The model under review builds one solid part; all positions refer to its coordinate system, in mm. Face numbers are marked on the shaded views. Round coordinates to 2 decimals unless told otherwise and drop trailing zeros. Order: outer loops, then holes, each group sorted by start corner. A loop starts at its lowest first (then second) coordinate and runs counter-clockwise, first axis right, second up. Notation, with made-up numbers: M 88.25,39 L 145.25,39 A7 ccw 145.25,52 Z; hole C 44,-40 d11. An arc over 180 degrees is marked long. Use a Markdown table: item, result. Add a question column.
1. Consider section B-B on z = 139. State the section outline as (x, y) points.
2. The part is to be moulded in two halves that separate along X. For the marked faces 1, 2, 3 and 4, say which applies: +X half, -X half, draft (parallel to the pull), parting line (faces both ways), or undercut.
3. Consider section A-A on z = 199. Count the separate pieces of the cut face and the enclosed holes in it, then the cut area to 3 significant figures.
4. Consider section D-D on y = 1.5. State the section outline as (x, z) points.
5. Consider section C-C on x = -63.5. State the section outline as (y, z) points (3 decimals).
6. To check wall thickness, follow probe 1 along Z at (x, y) = (88.9, -92.5); probe 2 along X at (y, z) = (-92, 209.55); probe 3 along X at (y, z) = (-84.5, 50.5). State the ranges of each line that lie inside material, in increasing order.
7. Insertion check: P1, Ø14, axis at x = -26.5, y = 83.5, coming from the +Z side; P2, Ø0.6, axis at x = -17.5, y = -88.5, coming from the +Z side; P3, Ø2.5, axis at x = 17, z = -1.5, coming from the -Y side; P4, Ø3, axis at x = -96.34, z = 209.55, coming from the +Y side. Each pin has a flat end and moves straight along its axis. Give the tip position at first contact, or say it passes through.
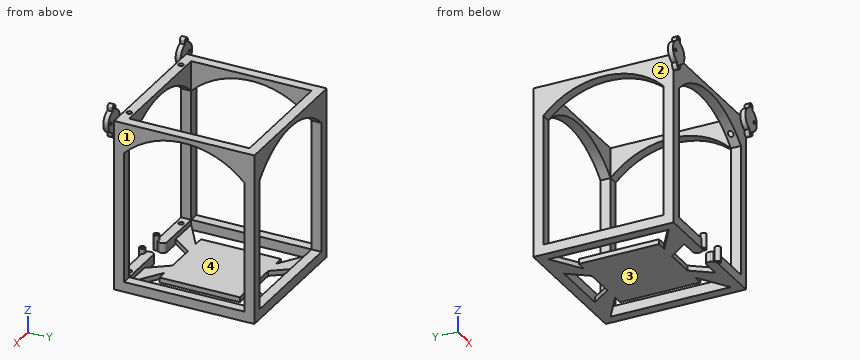
from build123d import *

# Parameters (mm, degrees)
F0_W      = 101.6
F0_H      = 101.6
F1_DEPTH  = 6.35
F2_W      = 12.7
F2_H      = 12.7
F3_DEPTH  = 88.9
F5_W      = 12.7
F5_H      = 12.7
F6_DEPTH  = 76.2
F9_W      = 38.1
F9_H      = 6.35
F8_W      = 19.05
F8_H      = 6.35
F14_W     = 12.7
F14_H     = 12.7
F15_DEPTH = 203.2
F17_DEPTH = 12.7
F20_DEPTH = 12.7
F22_R     = 3.175
F23_DEPTH = 209.55
F24_R     = 1.905
F24_R_2   = 1.778
F25_DEPTH = 19.05
F27_DEPTH = 25.4
F28_R     = 5.08
F29_R     = 1.778
F29_R_2   = 1.905
F30_DEPTH = 6.35


# Not quite as in the source:
# - a feature of the source that left no trace in its solid (it failed there, or was rolled back) is left out


with BuildPart() as f1:
    # F0 (on Top) → F1 (new body)
    with BuildSketch(Plane.XY):
        Rectangle(F0_W, F0_H)
    extrude(amount=-F1_DEPTH)



with BuildPart() as f3:
    # F2 (on Right) → F3 (new body, symmetric)
    with BuildSketch(Plane.YZ):
        with Locations((-82.55, 0)):
            Rectangle(F2_W, F2_H)
    extrude(amount=F3_DEPTH, both=True)


with BuildPart() as f4_1:
    # F4: instance of F3
    add(f3.part.mirror(Plane.XZ))


with BuildPart() as f3_1:
    add(f3.part)

    add(f4_1.part)  # F6 merges F4_1
    # F5 (on Front) → F6 (join, symmetric)
    with BuildSketch(Plane.XZ):
        with Locations((82.55, 0)):
            Rectangle(F5_W, F5_H)
    extrude(amount=F6_DEPTH, both=True)


with BuildPart() as f7_1:
    # F7: instance of F3
    add(f3_1.part.mirror(Plane.YZ))


with BuildPart() as f1_1:
    add(f1.part)

    add(f3_1.part)  # F10 merges F3

    add(f7_1.part)  # F10 merges F7_1
    # F9 (on face) → F10 section 0
    with BuildSketch(Plane(origin=(0, -76.2, 0), x_dir=(-1, 0, 0), z_dir=(0, 1, 0))):
        with Locations((57.15, -3.175)):
            Rectangle(F9_W, F9_H)
    # F8 (on face) → F10 section 1
    with BuildSketch(Plane.XZ.offset(50.8)):
        with Locations((-28.575, -3.175)):
            Rectangle(F8_W, F8_H)
    loft()


with BuildPart() as f11_1:
    # F11: instance of F1
    add(f1_1.part.mirror(Plane.YZ))


with BuildPart() as f12_1:
    # F12: instance of F11_1
    add(f11_1.part.mirror(Plane.XZ))


with BuildPart() as f12_2:
    # F12: instance of F1
    add(f1_1.part.mirror(Plane.XZ))


with BuildPart() as f1_2:
    add(f1_1.part)

    # F13: union F12_2, F11_1, F12_1
    add(f12_2.part)
    add(f11_1.part)
    add(f12_1.part)

    # F14 (on face) → F15 (join)
    with BuildSketch(Plane.XY.offset(6.35)):
        with Locations((-82.55, 82.55)):
            Rectangle(F14_W, F14_H)
        with Locations((82.55, 82.55)):
            Rectangle(F14_W, F14_H)
        with Locations((82.55, -82.55)):
            Rectangle(F14_W, F14_H)
        with Locations((-82.55, -82.55)):
            Rectangle(F14_W, F14_H)
    extrude(amount=F15_DEPTH)

    # F16 (on face) → F17 (join)
    with BuildSketch(Plane(origin=(-88.9, 0, 0), x_dir=(0, -1, 0), z_dir=(-1, 0, 0))):
        with BuildLine():
            ThreePointArc((-76.2, 171.45), (0, 203.2), (76.2, 171.45))
            Line((76.2, 171.45), (76.2, 209.55))
            Line((76.2, 209.55), (-76.2, 209.55))
            Line((-76.2, 209.55), (-76.2, 171.45))
        make_face()
    extrude(amount=-F17_DEPTH)

    # F18: F1 across plane


with BuildPart() as f1_3:
    add(f1_2.part)
    add(f1_2.part.mirror(Plane.YZ))

    # F19 (on face) → F20 (join)
    with BuildSketch(Plane(origin=(0, 88.9, 0), x_dir=(-1, 0, 0), z_dir=(0, 1, 0))):
        with BuildLine():
            ThreePointArc((-76.2, 171.45), (0, 203.2), (76.2, 171.45))
            Line((76.2, 171.45), (76.2, 209.55))
            Line((76.2, 209.55), (-76.2, 209.55))
            Line((-76.2, 209.55), (-76.2, 171.45))
        make_face()
    extrude(amount=-F20_DEPTH)

    # F21: F1 across plane


with BuildPart() as f1_4:
    add(f1_3.part)
    add(f1_3.part.mirror(Plane.XZ))

    # F22 (on face) → F23 (cut)
    with BuildSketch(Plane.XY.offset(209.55)):
        with Locations((-63.5, -82.55)):
            Circle(F22_R)
        with Locations((63.5, -82.55)):
            Circle(F22_R)
    extrude(amount=-F23_DEPTH, mode=Mode.SUBTRACT)

    # F24 (on face) → F25 (join)
    with BuildSketch(Plane(origin=(0, 0, -6.35), x_dir=(1, 0, 0), z_dir=(0, 0, -1))):
        with BuildLine():
            Line((17.45107, 93.48597), (13.5244245713, 93.48597))
            ThreePointArc((13.5244245713, 93.48597), (0, 103.95585), (-13.5244245713, 93.48597))
            Line((-13.5244245713, 93.48597), (-17.45107, 93.48597))
            ThreePointArc((-17.45107, 93.48597), (-20.95119, 89.98585), (-17.45107, 86.48573))
            Line((-17.45107, 86.48573), (-13.5244245713, 86.48573))
            ThreePointArc((-13.5244245713, 86.48573), (0, 76.01585), (13.5244245713, 86.48573))
            Line((13.5244245713, 86.48573), (17.45107, 86.48573))
            ThreePointArc((17.45107, 86.48573), (20.95119, 89.98585), (17.45107, 93.48597))
        make_face()
        with Locations((0, 82.55)):
            Circle(F24_R, mode=Mode.SUBTRACT)
        with Locations((-17.45107, 89.98585)):
            Circle(F24_R_2, mode=Mode.SUBTRACT)
        with Locations((17.45107, 89.98585)):
            Circle(F24_R_2, mode=Mode.SUBTRACT)
    extrude(amount=-F25_DEPTH)

    # F26 (on face) → F27 (cut)
    with BuildSketch(Plane.XY.offset(12.7)):
        with BuildLine():
            ThreePointArc((-17.45107, -86.48573), (-15.0942845585, -87.3981092098), (-13.9661895841, -89.6595855349))
            ThreePointArc((-13.9661895841, -89.6595855349), (-13.97, -89.98585), (-13.9661895841, -90.3121144651))
            ThreePointArc((-13.9661895841, -90.3121144651), (-15.0942845585, -92.5735907902), (-17.45107, -93.48597))
            Line((-17.45107, -93.48597), (-13.5244245713, -93.48597))
            ThreePointArc((-13.5244245713, -93.48597), (0, -103.95585), (13.5244245713, -93.48597))
            Line((13.5244245713, -93.48597), (17.45107, -93.48597))
            ThreePointArc((17.45107, -93.48597), (13.95095, -89.98585), (17.45107, -86.48573))
            Line((17.45107, -86.48573), (13.5244245713, -86.48573))
            ThreePointArc((13.5244245713, -86.48573), (0, -76.01585), (-13.5244245713, -86.48573))
            Line((-13.5244245713, -86.48573), (-17.45107, -86.48573))
        make_face()
    extrude(amount=-F27_DEPTH, mode=Mode.SUBTRACT)

    # F28
    f28_edges = [f1_4.edges().sort_by_distance(p)[0] for p in [
        (2.260805, -76.2, 0),
        (-2.260805, -76.2, 0),
    ]]
    fillet(f28_edges, radius=F28_R)

    # F29 (on face) → F30 (join)
    with BuildSketch(Plane.XZ.offset(88.9)):
        with BuildLine():
            Line((-85.39988, 192.09893), (-85.39988, 196.0255754287))
            ThreePointArc((-85.39988, 196.0255754287), (-74.93, 209.55), (-85.39988, 223.0744245713))
            Line((-85.39988, 223.0744245713), (-85.39988, 227.00107))
            ThreePointArc((-85.39988, 227.00107), (-88.9, 230.50119), (-92.40012, 227.00107))
            Line((-92.40012, 227.00107), (-92.40012, 223.0744245713))
            ThreePointArc((-92.40012, 223.0744245713), (-102.87, 209.55), (-92.40012, 196.0255754287))
            Line((-92.40012, 196.0255754287), (-92.40012, 192.09893))
            ThreePointArc((-92.40012, 192.09893), (-88.9, 188.59881), (-85.39988, 192.09893))
        make_face()
        with Locations((-88.9, 192.09893)):
            Circle(F29_R, mode=Mode.SUBTRACT)
        with Locations((-96.33585, 209.55)):
            Circle(F29_R_2, mode=Mode.SUBTRACT)
        with Locations((-88.9, 227.00107)):
            Circle(F29_R, mode=Mode.SUBTRACT)
        with BuildLine():
            Line((85.39988, 227.00107), (85.39988, 223.0744245713))
            ThreePointArc((85.39988, 223.0744245713), (74.93, 209.55), (85.39988, 196.0255754287))
            Line((85.39988, 196.0255754287), (85.39988, 192.09893))
            ThreePointArc((85.39988, 192.09893), (88.9, 188.59881), (92.40012, 192.09893))
            Line((92.40012, 192.09893), (92.40012, 196.0255754287))
            ThreePointArc((92.40012, 196.0255754287), (102.87, 209.55), (92.40012, 223.0744245713))
            Line((92.40012, 223.0744245713), (92.40012, 227.00107))
            ThreePointArc((92.40012, 227.00107), (88.9, 230.50119), (85.39988, 227.00107))
        make_face()
        with Locations((88.9, 192.09893)):
            Circle(F29_R, mode=Mode.SUBTRACT)
        with Locations((96.33585, 209.55)):
            Circle(F29_R_2, mode=Mode.SUBTRACT)
        with Locations((88.9, 227.00107)):
            Circle(F29_R, mode=Mode.SUBTRACT)
    extrude(amount=F30_DEPTH)


solid = f1_4.part
Answer block:
| question | item | result |
|---|---|---|
| 1 | outline | M -88.9,-88.9 L -76.2,-88.9 L -76.2,-76.2 L -88.9,-76.2 Z; M -88.9,76.2 L -76.2,76.2 L -76.2,88.9 L -88.9,88.9 Z; M 76.2,-88.9 L 88.9,-88.9 L 88.9,-76.2 L 76.2,-76.2 Z; M 76.2,76.2 L 88.9,76.2 L 88.9,88.9 L 76.2,88.9 Z |
| 2 | face 1 | +X half |
| 2 | face 2 | -X half |
| 2 | face 3 | draft |
| 2 | face 4 | undercut |
| 3 | separate pieces | 4 |
| 3 | enclosed holes | 2 |
| 3 | area | 5,540 mm^2 |
| 4 | outline | M -88.9,-6.35 L -76.2,-6.35 L -76.2,6.35 L -88.9,6.35 Z; M -88.9,203.19 L -76.2,203.19 L -76.2,209.55 L -88.9,209.55 Z; M -50.8,-6.35 L 50.8,-6.35 L 50.8,0 L -50.8,0 Z; M 76.2,-6.35 L 88.9,-6.35 L 88.9,6.35 L 76.2,6.35 Z; M 76.2,203.19 L 88.9,203.19 L 88.9,209.55 L 76.2,209.55 Z |
| 5 | outline | M -88.9,-6.35 L -67.733,-6.35 L -67.733,0 L -76.2,0 L -76.2,6.35 L -79.375,6.35 L -79.375,0 L -85.725,0 L -85.725,6.35 L -88.9,6.35 Z; M -88.9,182.397 L -85.725,182.397 L -85.725,209.55 L -88.9,209.55 Z; M -79.375,182.397 L -76.2,182.397 L -76.2,209.55 L -79.375,209.55 Z; M 67.733,-6.35 L 88.9,-6.35 L 88.9,6.35 L 76.2,6.35 L 76.2,0 L 67.733,0 Z; M 76.2,182.397 L 88.9,182.397 L 88.9,209.55 L 76.2,209.55 Z |
| 6 | probe 1 | 188.6 to 190.32, 193.88 to 225.22, 228.78 to 230.5 |
| 6 | probe 2 | -102.87 to -98.24, -94.43 to -74.93, 74.93 to 94.43, 98.24 to 102.87 |
| 6 | probe 3 | -88.9 to -76.2, 76.2 to 88.9 |
| 7 | P1 | z = 209.55 |
| 7 | P2 | z = 209.55 |
| 7 | P3 | y = -93.49 |
| 7 | P4 | through |
